Check sheet for the modelled part. Datum: model origin and axes. Units: mm. Face numbers are marked on the shaded views. A direction names the side the tool comes from. Round coordinates to 2 decimals unless told otherwise and drop trailing zeros. Order: outer loops, then holes, each group sorted by start corner. A loop starts at its lowest first (then second) coordinate and runs counter-clockwise, first axis right, second up. Notation, with made-up numbers: (45.25, 75) -> (76.25, 75) arc R21 cw to (76.25, 98) -> close; hole circle Ø1 at (-26.75, 11.5). An arc over 180 degrees is marked (long way). Answer in a Markdown table with one row per item.
from build123d import *

# Parameters (mm, degrees)
SKETCH_1_W          = 20
SKETCH_1_H          = 20
SKETCH_1_W_2        = 18
SKETCH_1_H_2        = 18
EXTRUDE_1_DEPTH     = 89
SKETCH_2_R          = 2
CUT_EXTRUDE_1_DEPTH = 94.386294498


with BuildPart() as part:
    # 草图1 → 拉伸-薄壁1 (new body)
    with BuildSketch(Plane.XY):
        with Locations((10, 10)):
            Rectangle(SKETCH_1_W, SKETCH_1_H)
        with Locations((10, 10)):
            Rectangle(SKETCH_1_W_2, SKETCH_1_H_2, mode=Mode.SUBTRACT)
    extrude(amount=EXTRUDE_1_DEPTH)

    # 草图2 → 切除-拉伸1 (cut, through all)
    with BuildSketch(Plane(origin=(0, 20, 0), x_dir=(1, 0, 0), z_dir=(0, 1, 0))):
        with Locations(Location((5, -5, 0), (0, 0, 270))):
            Circle(SKETCH_2_R)
        with Locations(Location((15, -5, 0), (0, 0, 270))):
            Circle(SKETCH_2_R)
        with Locations(Location((5, -25, 0), (0, 0, 270))):
            Circle(SKETCH_2_R)
        with Locations(Location((15, -25, 0), (0, 0, 270))):
            Circle(SKETCH_2_R)
        with Locations(Location((15, -84, 0), (0, 0, 270))):
            Circle(SKETCH_2_R)
        with Locations(Location((15, -69, 0), (0, 0, 270))):
            Circle(SKETCH_2_R)
        with Locations(Location((15, -54, 0), (0, 0, 270))):
            Circle(SKETCH_2_R)
    extrude(amount=-CUT_EXTRUDE_1_DEPTH, mode=Mode.SUBTRACT)


solid = part.part
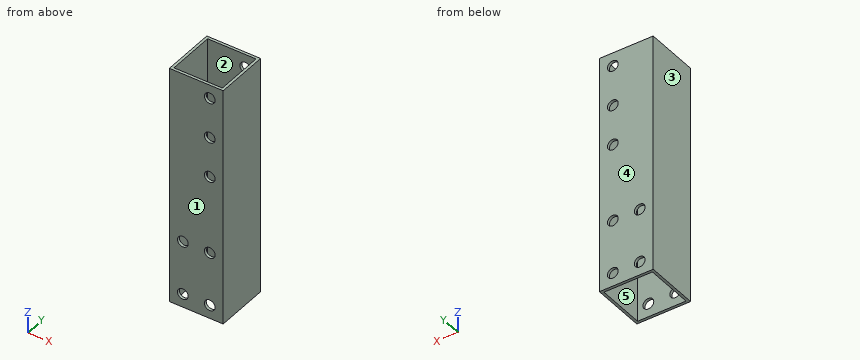
Item 1: Mould release check, pull along X, two halves, no side actions. Record for the marked faces 3, 4 and 5: pulls with the +X half, pulls with the -X half, needs draft (parallel to the pull), parting line crosses it, or undercut.
Result sheet:
| item | result |
|---|---|
| face 3 | pulls with the -X half |
| face 4 | needs draft |
| face 5 | undercut |
Item 2: Cross-section at D-D (z = 5). Record the boundary of the cut face in (x, y), and give its area (3 significant figures).
Result sheet:
| item | result |
|---|---|
| outline | (0, 0) -> (3, 0) -> (3, 1) -> (1, 1) -> (1, 19) -> (3, 19) -> (3, 20) -> (0, 20) -> close; (7, 0) -> (13, 0) -> (13, 1) -> (7, 1) -> close; (7, 19) -> (13, 19) -> (13, 20) -> (7, 20) -> close; (17, 0) -> (20, 0) -> (20, 20) -> (17, 20) -> (17, 19) -> (19, 19) -> (19, 1) -> (17, 1) -> close |
| area | 60.0 mm^2 |
Item 3: Cross-section at B-B (y = 15.75). Record the boundary of the cut face in (x, z).
Result sheet:
| item | result |
|---|---|
| outline | (0, 0) -> (1, 0) -> (1, 89) -> (0, 89) -> close; (19, 0) -> (20, 0) -> (20, 89) -> (19, 89) -> close |
Item 4: Depth check by flat-ended pin: P1, Ø5, axis at x = 15, z = 54, coming from the -Y side; P2, Ø3, axis at x = 5, z = 25, coming from the -Y side. Enter the tip coordinate at first touch or a pass-through.
Result sheet:
| item | result |
|---|---|
| P1 | stops at y = 0 |
| P2 | passes through |
Item 5: Set-up check for the marked faces 1 and 2: record each of +Z, -Z, +X, -X, +Y, -Y from which the full face is reachable in a straight line by a thin tool's end or side.
Result sheet:
| item | result |
|---|---|
| face 1 | +Z, -Z, +X, -X, -Y |
| face 2 | +Z, -Z |
Item 6: Scan lines: line 1 (X direction, y = 19.6, z = 5); line 2 (Y direction, x = 13.5, z = 26.5); line 3 (X direction, y = 0.75, z = 84). Record each from-to range of solid material in increasing order. Write a range as [from, to].
Result sheet:
| item | result |
|---|---|
| line 1 | x = [0, 3], [7, 13], [17, 20] |
| line 2 | y = [0, 1], [19, 20] |
| line 3 | x = [0, 13], [17, 20] |
Item 7: Cross-section at A-A (z = 84). Record the boundary of the cut face in (x, y), and give its area (3 significant figures).
Result sheet:
| item | result |
|---|---|
| outline | (0, 0) -> (13, 0) -> (13, 1) -> (1, 1) -> (1, 19) -> (13, 19) -> (13, 20) -> (0, 20) -> close; (17, 0) -> (20, 0) -> (20, 20) -> (17, 20) -> (17, 19) -> (19, 19) -> (19, 1) -> (17, 1) -> close |
| area | 68.0 mm^2 |
